```python
from build123d import *

# Parameters (mm, degrees)
F1_R     = 25
F2_DEPTH = 2
F0_R     = 3.9
F3_DEPTH = 18
F4_R     = 2
F0_R_2   = 3
F5_DEPTH = 2


with BuildPart() as f2:
    # F1 (on Top) → F2 (new body)
    with BuildSketch(Plane.XY):
        Circle(F1_R)
    extrude(amount=-F2_DEPTH)

    # F0 (on Top) → F3 (join)
    with BuildSketch(Plane.XY):
        with Locations((-12.9903810568, -7.5)):
            Circle(F0_R)
        with Locations((0, 15)):
            Circle(F0_R)
        with Locations((12.9903810568, -7.5)):
            Circle(F0_R)
    extrude(amount=F3_DEPTH)

    # F4
    f4_edges = [f2.edges().sort_by_distance(p)[0] for p in [
        (9.090381, -7.5, 0),
        (-3.9, 15, 0),
        (-16.890381, -7.5, 0),
    ]]
    fillet(f4_edges, radius=F4_R)

    # F0 (on Top) → F5 (cut)
    with BuildSketch(Plane.XY):
        with Locations((12.9903810568, 7.5)):
            Circle(F0_R_2)
        with Locations((-12.9903810568, 7.5)):
            Circle(F0_R_2)
        with Locations((0, -15)):
            Circle(F0_R_2)
    extrude(amount=-F5_DEPTH, mode=Mode.SUBTRACT)


solid = f2.part
```
The model under review builds one solid part; all positions refer to its coordinate system, in mm. A direction names the side the tool comes from. Round coordinates to 2 decimals unless told otherwise and drop trailing zeros. Order: outer loops, then holes, each group sorted by start corner. A loop starts at its lowest first (then second) coordinate and runs counter-clockwise, first axis right, second up. Notation, with made-up numbers: M 55,62.5 L 60,62.5 A25 ccw 60,78.5 Z; hole C 64.5,74.25 d1. An arc over 180 degrees is marked long. Use a Markdown table: item, result.
1) Wall thickness on line 1 along Z through (x, y) = (-0.5, -19.5); line 2 along X through (y, z) = (-14.5, -0.5); line 3 along Y through (x, z) = (-14, -1) (3 decimals): over which ranges is each line inside the solid? List them lowest first. Write a range as [from, to].
Report:
| item | result |
|---|---|
| line 1 | [-2, 0] |
| line 2 | [-20.37, -2.96], [2.96, 20.37] |
| line 3 | [-20.712, 4.675], [10.325, 20.712] |
2) Consider section A-A (y = -15). Write out the cut boundary in (x, z).
Report:
| item | result |
|---|---|
| outline | M -20,-2 L -3,-2 L -3,0 L -20,0 Z; M 3,-2 L 20,-2 L 20,0 L 3,0 Z |
3) Draft analysis for pull direction X (two halves, no side actions). For faces 1 (the face through (-13, -7, 18)), 2 (the face through (-10.2, 6.4, -1)), 3 (the face through (23.846, 7.509, -0.986)), 4 (the face through (15.76, 6.35, -0.99)), state which applies: released by +X, released by -X, zero draft, split by the parting line, or undercut.
Report:
| item | result |
|---|---|
| face 1 | zero draft |
| face 2 | undercut |
| face 3 | split by the parting line |
| face 4 | undercut |
4) Consider section B-B (x = 0). Write out the cut boundary in (y, z).
Report:
| item | result |
|---|---|
| outline | M -25,-2 L -18,-2 L -18,0 L -25,0 Z; M -12,-2 L 25,-2 L 25,0 L 20.9,0 A2 cw 18.9,2 L 18.9,18 L 11.1,18 L 11.1,2 A2 cw 9.1,0 L -12,0 Z |
5) Insertion check: pin 1 (5.5 mm diameter, centred on x = 0, y = -15, fed in from -Z); pin 2 (10 mm diameter, centred on x = -9, z = 1.5, fed in from -Y); pin 3 (1.5 mm diameter, centred on x = 14, y = -2, fed in from +Z); pin 4 (12 mm diameter, centred on x = 17, z = 5.5, fed in from -Y). Each pin has a flat end and moves straight along its axis. Give the tip position at first contact, or say it passes through.
Report:
| item | result |
|---|---|
| pin 1 | through |
| pin 2 | y = -24.64 |
| pin 3 | z = 0.3 |
| pin 4 | y = -20.29 |
6) Consider section D-D (z = 7.5). Write out the cut boundary in (x, y), then the cut area to 3 significant figures.
Report:
| item | result |
|---|---|
| outline | C -12.99,-7.5 d7.8; C 0,15 d7.8; C 12.99,-7.5 d7.8 |
| area | 143 mm^2 |
7) Consider section C-C (y = 15). Write out the cut boundary in (x, z).
Report:
| item | result |
|---|---|
| outline | M -20,-2 L 20,-2 L 20,0 L 5.9,0 A2 cw 3.9,2 L 3.9,18 L -3.9,18 L -3.9,2 A2 cw -5.9,0 L -20,0 Z |
8) Tool access review of faces 5 (the face through (13, -7, 18)), 6 (the face through (-0.508, 18.867, 9.888)): name each direction out of +Z, -Z, +X, -X, +Y, -Y from which nothing blocks a thin tool from reaching the whole face with its end or side.
Report:
| item | result |
|---|---|
| face 5 | +Z, +X, -X, +Y, -Y |
| face 6 | +Z |
